Autodesk Inventor part; units mm, degrees
ref_plane "YZ Plane" through (0, 0, 0) normal (1, 0, 0) x (0, 1, 0)
ref_plane "XZ Plane" through (0, 0, 0) normal (0, 1, 0) x (-1, 0, 0)
ref_plane "XY Plane" through (0, 0, 0) normal (0, 0, 1) x (1, 0, 0)
sketch "Эскиз1" plane through (0, 0, 0) normal (0, 0, 1) x (1, 0, 0)
  line L0 (0, 0) -> (350.66, 0)
  line L1 (350.66, 0) -> (350.66, 205.25)
  line L2 (350.66, 205.25) -> (0, 205.25)
  line L3 (0, 205.25) -> (0, 0)
  line L4 (3.25, 202) -> (347.41, 202)
  line L5 (347.41, 202) -> (347.41, 8.5)
  line L6 (347.41, 8.5) -> (3.25, 8.5)
  line L7 (3.25, 8.5) -> (3.25, 202)
  line L8 (35.18, 0) -> (315.48, 0)
  line L9 (315.48, 0) -> (315.48, -11)
  line L10 (315.48, -11) -> (35.18, -11)
  line L11 (35.18, -11) -> (35.18, 0)
  line L12 (175.33, 8.5) -> (175.33, 37.7602)
  point P0 (175.33, 202)
  point P1 (175.33, 205.25)
  point P2 (175.33, -11)
  dimension "d0" = 350.66
  dimension "d1" = 205.25
  dimension "d2" = 344.16
  dimension "d3" = 193.5
  dimension "d4" = 3.25
  dimension "d5" = 8.5
  dimension "d6" = 3.25
  dimension "d7" = 216.25
  dimension "d9" = 280.3
  dimension "d28" = 35.18
extrude "Выдавливание1" add sketch "Эскиз1" along normal blind 3.2
sketch "Эскиз2" plane through (0, 0, 3.2) normal (0, 0, 1) x (1, 0, 0)
  line L0 (0, 0) -> (35.18, 0)
  line L1 (35.18, 0) -> (35.18, -11)
  line L2 (35.18, -11) -> (315.48, -11)
  line L3 (315.48, -11) -> (315.48, 0)
  line L4 (315.48, 0) -> (350.66, 0)
  line L5 (350.66, 0) -> (350.66, 205.25)
  line L6 (350.66, 205.25) -> (0, 205.25)
  line L7 (0, 205.25) -> (0, 0)
  line L8 (347.41, 202) -> (347.41, 8.5)
  line L9 (347.41, 8.5) -> (3.25, 8.5)
  line L10 (3.25, 8.5) -> (3.25, 202)
  line L11 (3.25, 202) -> (347.41, 202)
extrude "Выдавливание2" add sketch "Эскиз2" against normal blind 3.4 contours L8 L9 L10 L11
sketch "Эскиз3" plane through (0, 0, 0) normal (0, 0, -1) x (-1, 0, 0)
  line L0 (0, 0) -> (-35.18, 0)
  line L1 (0, 205.25) -> (0, 0)
  line L2 (-350.66, 205.25) -> (0, 205.25)
  line L3 (-350.66, 0) -> (-350.66, 205.25)
  line L4 (-315.48, 0) -> (-350.66, 0)
  line L5 (-315.48, -11) -> (-315.48, 0)
  line L6 (-35.18, -11) -> (-315.48, -11)
  line L7 (-35.18, 0) -> (-35.18, -11)
  line L8 (-347.41, 202) -> (-347.41, 8.5)
  line L9 (-3.25, 202) -> (-347.41, 202)
  line L10 (-3.25, 8.5) -> (-3.25, 202)
  line L11 (-347.41, 8.5) -> (-3.25, 8.5)
  line L12 (-175.33, -11) -> (-175.33, 1.1845)
  line L13 (-235.57, 5.5) -> (-210.63, 5.5)
  line L14 (-210.63, 5.5) -> (-210.63, 3.5)
  line L15 (-210.63, 3.5) -> (-235.57, 3.5)
  line L16 (-235.57, 3.5) -> (-235.57, 5.5)
  line L17 (-319.31, 5.5) -> (-294.37, 5.5)
  line L18 (-294.37, 5.5) -> (-294.37, 3.5)
  line L19 (-294.37, 3.5) -> (-319.31, 3.5)
  line L20 (-319.31, 3.5) -> (-319.31, 5.5)
  line L21 (-115.09, 5.5) -> (-140.03, 5.5)
  line L22 (-140.03, 5.5) -> (-140.03, 3.5)
  line L23 (-140.03, 3.5) -> (-115.09, 3.5)
  line L24 (-115.09, 3.5) -> (-115.09, 5.5)
  line L25 (-31.35, 5.5) -> (-56.29, 5.5)
  line L26 (-56.29, 5.5) -> (-56.29, 3.5)
  line L27 (-56.29, 3.5) -> (-31.35, 3.5)
  line L28 (-31.35, 3.5) -> (-31.35, 5.5)
  point P0 (-294.37, 4.5)
  point P1 (-235.57, 4.5)
  point P2 (-56.29, 4.5)
  point P3 (-115.09, 4.5)
  dimension "d14" = 24.94
  dimension "d15" = 35.3
  dimension "d16" = 3
  dimension "d17" = 2
  dimension "d18" = 2
  dimension "d19" = 24.94
  dimension "d20" = 58.8
extrude "Выдавливание3" cut sketch "Эскиз3" against normal blind 1 contours L13 L14 L15 L16 | L17 L18 L19 L20 | L24 L23 L22 L21 | L28 L27 L26 L25
sketch "Эскиз5" plane through (0, 0, 3.2) normal (0, 0, 1) x (1, 0, 0)
  line L0 (0, 0) -> (35.18, 0)
  line L1 (35.18, 0) -> (35.18, -11)
  line L2 (35.18, -11) -> (315.48, -11)
  line L3 (315.48, -11) -> (315.48, 0)
  line L4 (315.48, 0) -> (350.66, 0)
  line L5 (350.66, 0) -> (350.66, 205.25)
  line L6 (350.66, 205.25) -> (0, 205.25)
  line L7 (0, 205.25) -> (0, 0)
  line L8 (205.66, -11) -> (240.66, -11)
  line L9 (240.66, -11) -> (240.66, 9)
  line L10 (240.66, 9) -> (205.66, 9)
  line L11 (205.66, 9) -> (205.66, -11)
  dimension "d23" = 110
  dimension "d24" = 20
  dimension "d25" = 35
extrude "Выдавливание4" cut sketch "Эскиз5" against normal blind 1 contours L11 L10 L9 L2
equation "\"d19\" = d14"
properties part number "Матрица от ноутбука 15.6 NV156FHM-N42ipt"
Geometry check sheet. Reference: the model listing, model coordinates, mm. Coordinates: 2 decimals unless noted, no trailing zeros. One line per item, written item: value. Start each with the question number.
(1) Material ranges on line 1 (Y direction, x = 28, z = 1.5); line 2 (Z direction, x = 327, y = 8), recorded low to high. Write a range as [from, to].
(2) Depth check by flat-ended pin: P1, Ø6, axis at x = 216, y = 2, coming from the +Z side; P2, Ø1.6, axis at x = 325, z = 2, coming from the -Y side. Enter the tip coordinate at first touch or a pass-through.
(3) Mould release check, pull along X, two halves, no side actions. Record for faces 1 (the flat face through (223, -1, 2.2)), 2 (the flat face through (173, 107, -0.2)): released by +X, released by -X, zero draft, split by the parting line, or undercut.
Results below:
1. line 1: y = [0, 205.25]
1. line 2: z = [0, 3.2]
2. P1: stops at z = 2.2
2. P2: stops at y = 0
3. face 1: undercut
3. face 2: zero draft
